Could you check a few things on this model? Use its own coordinates, in mm. Face numbers are marked on the shaded views. A direction names the side the tool comes from. Coordinates: 2 decimals unless noted, no trailing zeros. Loops run counter-clockwise (first coordinate to the right, second up) from the corner with the lowest first, then second, coordinate; pieces in that order, holes last. Notation, with made-up numbers: (-25.5, 34) -> (33.5, 34) arc R28 cw to (33.5, 59) -> close; hole circle Ø8 at (67, 80.5). An arc over 180 degrees is marked (long way). One line per question, with ' | ' between items. Start each with the question number.
(1) Which directions (+Z, -Z, +X, -X, +Y, -Y) give clear straight access to the entire face, cutting with the end or side of a thin tool? Please do the marked faces 1, 2 and 3.
(2) If I drill on line 1 along Y through (x, z) = (-34.5, -0.75); line 2 along Z through (x, y) = (-8.5, -3), over which ranges is the centre line in solid material (lowest first)?
(3) I'm going to push flat-ended pins straight in: pin 1 Ø12 at (x, z) = (-2.5, -8.5) entering from +Y; pin 2 Ø1.5 at (x, z) = (-25.5, -20.5) entering from -Y. Where does each tip first touch, or does it pass through?
(4) Suppose I cut it at A-A (x = -34). Please give me the cut outline in (y, z), plus the area to 3 significant figures.
(5) Suppose I cut it at B-B (z = -18.25). Please give me the cut outline in (x, y).
```python
from build123d import *

# Parameters (mm, degrees)
SKETCH_1_W             = 44.4
SKETCH_1_H             = 23.4
EXTRUDE_1_DEPTH        = 28
SKETCH_2_R             = 2.5
EXTRUDE_2_DEPTH        = 5
PATTERN_LINEAR_1_COUNT = 2
PATTERN_LINEAR_1_PITCH = 33


with BuildPart() as part:
    # 草圖1 → 填料-伸長1 (new body)
    with BuildSketch(Plane(origin=(0, 0, 0), x_dir=(1, 0, 0), z_dir=(0, 1, 0))):
        with Locations((-19.947783251, 11.493103448)):
            Rectangle(SKETCH_1_W, SKETCH_1_H)
    extrude(amount=EXTRUDE_1_DEPTH)

    # 草圖2 → 填料-伸長2 (add)
    with BuildSketch(Plane(origin=(0, 0, 0), x_dir=(1, 0, 0), z_dir=(0, 1, 0))):
        with Locations((-7.747783251, 11.493103448)):
            Circle(SKETCH_2_R)
    extrude_2 = extrude(amount=-EXTRUDE_2_DEPTH)

    # 直線複製排列1: 填料-伸長2 ×2
    with Locations(*[(0, i * PATTERN_LINEAR_1_PITCH, 0) for i in range(1, PATTERN_LINEAR_1_COUNT)]):
        add(extrude_2)


solid = part.part
```
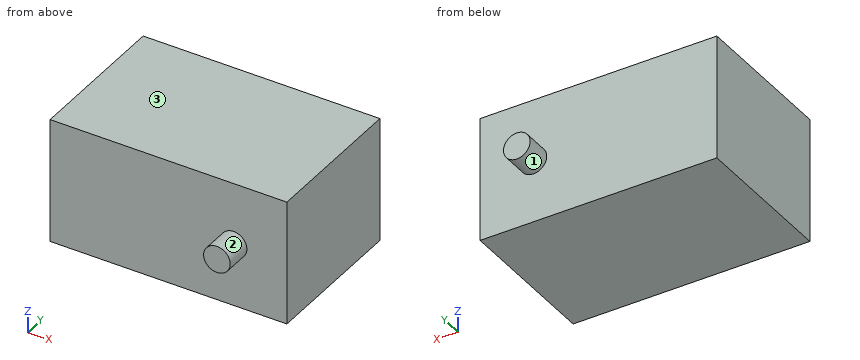
Checks:
1) face 1: +Y | face 2: -Y | face 3: +Z, +X, -X, +Y, -Y
2) line 1: y = 0 to 28 | line 2: z = -13.88 to -9.11
3) pin 1: stops at y = 33 | pin 2: stops at y = 0
4) outline: (0, -23.19) -> (28, -23.19) -> (28, 0.21) -> (0, 0.21) -> close | area: 655 mm^2
5) outline: (-42.15, 0) -> (2.25, 0) -> (2.25, 28) -> (-42.15, 28) -> close
